Geometry: final body of the model. Coordinates: model frame, mm. A direction names the side the tool comes from. Coordinates: 2 decimals unless noted, no trailing zeros. Order: outer loops, then holes, each group sorted by start corner. A loop starts at its lowest first (then second) coordinate and runs counter-clockwise, first axis right, second up. Notation, with made-up numbers: (14, 60.25) -> (69, 60.25) arc R8 cw to (69, 75.25) -> close; hole circle Ø9 at (31.25, 46.5). An arc over 180 degrees is marked (long way). Use one line per item in the form item = value.
```python
from build123d import *

# Parameters (mm, degrees)
SKETCH1_R               = 13.335
SKETCH1_R_2             = 10.4648
BOSS_EXTRUDE1_DEPTH     = 33.02
SKETCH2_W               = 6.35
SKETCH2_H               = 13.335
CUT_EXTRUDE1_DEPTH      = 14.335
CUT_EXTRUDE1_DEPTH_BACK = 14.335


with BuildPart() as part:
    # Sketch1 → Boss-Extrude1 (new body)
    with BuildSketch(Plane(origin=(0, 0, 0), x_dir=(0, 0, -1), z_dir=(1, 0, 0))):
        Circle(SKETCH1_R)
        Circle(SKETCH1_R_2, mode=Mode.SUBTRACT)
    extrude(amount=BOSS_EXTRUDE1_DEPTH)

    # Sketch2 → Cut-Extrude1 (cut, two sides)
    with BuildSketch(Plane.XY) as cut_extrude1_sk:
        with Locations((22.225, -6.6675)):
            Rectangle(SKETCH2_W, SKETCH2_H)
    extrude(amount=CUT_EXTRUDE1_DEPTH, mode=Mode.SUBTRACT)
    extrude(cut_extrude1_sk.sketch, amount=-CUT_EXTRUDE1_DEPTH_BACK, mode=Mode.SUBTRACT)


solid = part.part
```
1) Section C-C, the plane x = 29. Output: boundary loops of the cut face in (y, z) (3 decimals).
Results found:
outline = circle Ø26.67 at (0, 0); hole circle Ø20.93 at (0, 0)
2) Contact query for flat-ended pins moving along their axis: P1, Ø6, axis at x = 19, z = 5.5, coming from the -Y side; P2, Ø1.4, axis at x = 22.5, z = 11.5, coming from the -Y side; P3, Ø8, axis at x = 3.5, z = -5, coming from the -Y side. Output: stop coordinate, or through.
Results found:
P1 = -13.1
P2 = 0
P3 = -13.3
3) Section B-B, the plane y = 8. Output: boundary loops of the cut face in (x, z), and give its area (3 significant figures).
Results found:
outline = (0, -10.67) -> (33.02, -10.67) -> (33.02, -6.75) -> (0, -6.75) -> close; (0, 6.75) -> (33.02, 6.75) -> (33.02, 10.67) -> (0, 10.67) -> close
area = 259 mm2
4) Section D-D, the plane y = -8.5. Output: boundary loops of the cut face in (x, z).
Results found:
outline = (0, -10.27) -> (19.05, -10.27) -> (19.05, -6.1) -> (0, -6.1) -> close; (0, 6.1) -> (19.05, 6.1) -> (19.05, 10.27) -> (0, 10.27) -> close; (25.4, -10.27) -> (33.02, -10.27) -> (33.02, -6.1) -> (25.4, -6.1) -> close; (25.4, 6.1) -> (33.02, 6.1) -> (33.02, 10.27) -> (25.4, 10.27) -> close
5) Access query for faces 5 (the flat face through (33.02, -7, 8)), 6 (the flat face through (22, 0, 12)). Directions: +Z, -Z, +X, -X, +Y, -Y. A direction counts if a zero-diameter tool reaches every point of the face in a straight line with its end or side. Return the directions, or none.
Results found:
face_5 = +Z, -Z, +X, +Y, -Y
face_6 = +Z, -Z, -Y
6) Material intervals for probe 1 along Y at (x, z) = (14.5, 0) (3 decimals); probe 2 along X at (y, z) = (-8.25, -6.75), sorted ascending. Write a range as from..to.
Results found:
probe_1 = -13.335..-10.465, 10.465..13.335
probe_2 = 0..19.05, 25.4..33.02
7) Pull-direction query (Y, two-part tool) for faces 1 (the flat face through (0, -7, 8)), 2 (the cylindrical face through (16.279, 10.376, 1.362)), 3 (the flat face through (22, 0, -12)), 4 (the cylindrical face through (16.28, 13.22, 1.74)); classes: released by +Y, released by -Y, zero draft, split by the parting line, or undercut.
Results found:
face_1 = zero draft
face_2 = undercut
face_3 = released by -Y
face_4 = split by the parting line
8) Section A-A, the plane z = 0. Output: boundary loops of the cut face in (x, y) (3 decimals), and give its area (3 significant figures).
Results found:
outline = (0, -13.335) -> (19.05, -13.335) -> (19.05, -10.465) -> (0, -10.465) -> close; (0, 10.465) -> (33.02, 10.465) -> (33.02, 13.335) -> (0, 13.335) -> close; (25.4, -13.335) -> (33.02, -13.335) -> (33.02, -10.465) -> (25.4, -10.465) -> close
area = 171 mm2
